```python
from build123d import *

# Parameters (mm, degrees)
SKETCH1_R           = 15
SKETCH1_R_2         = 3
BOSS_EXTRUDE1_DEPTH = 3
SKETCH2_W           = 5
SKETCH2_H           = 3
SKETCH2_W_2         = 3
SKETCH2_H_2         = 5
CUT_EXTRUDE1_DEPTH  = 3


with BuildPart() as part:
    # Sketch1 → Boss-Extrude1 (new body)
    with BuildSketch(Plane.XY):
        Circle(SKETCH1_R)
        Circle(SKETCH1_R_2, mode=Mode.SUBTRACT)
    extrude(amount=BOSS_EXTRUDE1_DEPTH)

    # Sketch2 → Cut-Extrude1 (cut)
    with BuildSketch(Plane.XY.offset(3)):
        with Locations((8.5, 0)):
            Rectangle(SKETCH2_W, SKETCH2_H)
        with Locations((0, 8.5)):
            Rectangle(SKETCH2_W_2, SKETCH2_H_2)
        with Locations((0, -8.5)):
            Rectangle(SKETCH2_W_2, SKETCH2_H_2)
        with Locations((-8.5, 0)):
            Rectangle(SKETCH2_W, SKETCH2_H)
    extrude(amount=-CUT_EXTRUDE1_DEPTH, mode=Mode.SUBTRACT)


solid = part.part
```
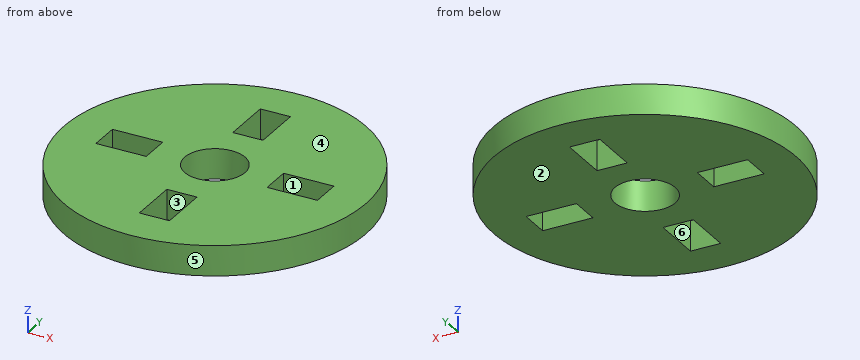
Here's how the part is built. I have some questions about the finished solid (model axes, mm). Face numbers are marked on the shaded views. A direction names the side the tool comes from. Coordinates: 2 decimals unless noted, no trailing zeros. Order: outer loops, then holes, each group sorted by start corner. A loop starts at its lowest first (then second) coordinate and runs counter-clockwise, first axis right, second up.
1) We'd pull the mould along X, two halves only. Please class the marked faces 3, 4, 5 and 6: +X half, -X half, draft (parallel to the pull), parting line (faces both ways), or undercut.
2) Imagine slicing it at D-D on x = -8.25. List the corners of the cut face in (y, z) for me.
3) Which directions (+Z, -Z, +X, -X, +Y, -Y) give clear straight access to the entire face, cutting with the end or side of a thin tool? Please do the marked faces 1 and 2.
4) I need wall thicknesses on line 1 (Y direction, x = 0, z = 2.35); line 2 (Y direction, x = -1.25, z = 1.85); line 3 (X direction, y = -7, z = 2.2). Which ranges of each line are inside material? Lowest first, please.
5) Imagine slicing it at C-C on y = -8. List the corners of the cut face in (x, z) for me, and give its area (3 significant figures).
6) Will these pins go through, and if not, where does the flat tip stop? pin 1 (0.9 mm diameter, centred on y = 8, z = 1, fed in from +X); pin 2 (0.9 mm diameter, centred on x = -9, z = 1, fed in from -Y); pin 3 (1 mm diameter, centred on x = 2.5, z = 2, fed in from +Y).
7) Imagine slicing it at A-A on y = 0. List the corners of the cut face in (x, z) for me.
Response values:
1. face 3: undercut
1. face 4: draft
1. face 5: parting line
1. face 6: undercut
2. outline: (-12.53, 0) - (-1.5, 0) - (-1.5, 3) - (-12.53, 3) - close; (1.5, 0) - (12.53, 0) - (12.53, 3) - (1.5, 3) - close
3. face 1: +Z, -Z
3. face 2: -Z, +X, -X, +Y, -Y
4. line 1: y = -15 to -11, -6 to -3, 3 to 6, 11 to 15
4. line 2: y = -14.95 to -11, -6 to -2.73, 2.73 to 6, 11 to 14.95
4. line 3: x = -13.27 to -1.5, 1.5 to 13.27
5. outline: (-12.69, 0) - (-1.5, 0) - (-1.5, 3) - (-12.69, 3) - close; (1.5, 0) - (12.69, 0) - (12.69, 3) - (1.5, 3) - close
5. area: 67.1 mm2
6. pin 1: stops at x = 12.96
6. pin 2: stops at y = -12.32
6. pin 3: stops at y = 14.87
7. outline: (-15, 0) - (-11, 0) - (-11, 3) - (-15, 3) - close; (-6, 0) - (-3, 0) - (-3, 3) - (-6, 3) - close; (3, 0) - (6, 0) - (6, 3) - (3, 3) - close; (11, 0) - (15, 0) - (15, 3) - (11, 3) - close
